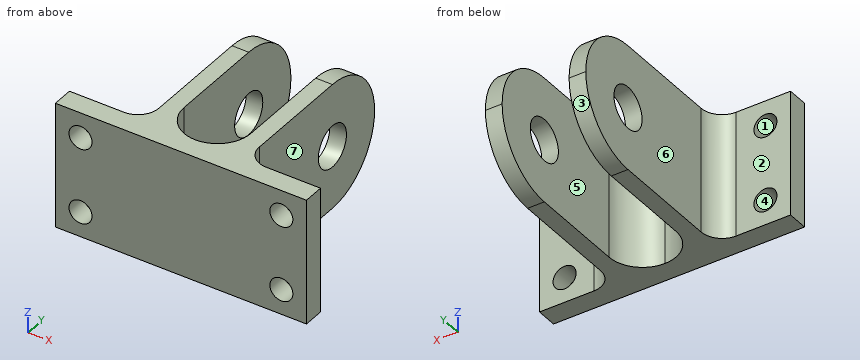
Autodesk Inventor part; units mm, degrees
ref_plane "YZ Plane" through (0, 0, 0) normal (1, 0, 0) x (0, 1, 0)
ref_plane "XZ Plane" through (0, 0, 0) normal (0, 1, 0) x (-1, 0, 0)
ref_plane "XY Plane" through (0, 0, 0) normal (0, 0, 1) x (1, 0, 0)
sketch "Sketch1" plane through (0, 0, 0) normal (0, 1, 0) x (-1, 0, 0)
  line L0 (-30, 15) -> (30, 15)
  line L1 (30, 15) -> (30, -15)
  line L2 (30, -15) -> (-30, -15)
  line L3 (-30, -15) -> (-30, 15)
  line L4 (-30, 15) -> (30, -15) construction
  line L5 (30, 15) -> (-30, -15) construction
  circle A0 centre (24, -9) radius 2.75
  circle A1 centre (24, 9) radius 2.75
  circle A2 centre (-24, 9) radius 2.75
  circle A3 centre (-24, -9) radius 2.75
  point P0 (0, 0)
  dimension "d0" = 60
  dimension "d1" = 30
  dimension "d2" = 5.5
  dimension "d3" = 5.5
  dimension "d4" = 5.5
  dimension "d5" = 5.5
  dimension "d6" = 6
  dimension "d7" = 6
  dimension "d8" = 6
  dimension "d9" = 6
  dimension "d10" = 6
  dimension "d11" = 6
  dimension "d12" = 6
  dimension "d13" = 6
extrude "Extrusion1" add sketch "Sketch1" along normal blind 5
sketch "Sketch2" plane through (0, 5, 0) normal (0, 1, 0) x (1, 0, 0)
  line L0 (8, -15) -> (-8, -15)
  line L1 (-8, -15) -> (-8, 15)
  line L2 (-8, 15) -> (8, 15)
  line L3 (8, 15) -> (8, -15)
  line L4 (8, -15) -> (-8, 15) construction
  line L5 (-8, -15) -> (8, 15) construction
  line L6 (-8, 15) -> (-12, 15)
  line L7 (-12, 15) -> (-12, -15)
  line L8 (-12, -15) -> (-8, -15)
  line L9 (-8, -15) -> (-8, 15)
  line L10 (8, -15) -> (12, -15)
  line L11 (12, -15) -> (12, 15)
  line L12 (12, 15) -> (8, 15)
  line L13 (8, 15) -> (8, -15)
  point P0 (0, 0)
  dimension "d16" = 16
  dimension "d17" = 30
  dimension "d18" = 4
  dimension "d19" = 30
  dimension "d20" = 4
extrude "Extrusion2" add sketch "Sketch2" along normal blind 46 contours L3 L12 L11 L10 | L8 L7 L6 L1
sketch "Sketch3" plane through (12, 5, 15) normal (1, 0, 0) x (0, 0, -1)
  circle A0 centre (15, 31) radius 5
  line L0 (30, 0) -> (30, 46)
  line L1 (30, -5) -> (0, -5)
  point P0 (15, -5)
  dimension "d23" = 10
  dimension "d24" = 15
  dimension "d25" = 36
extrude "Extrusion3" cut sketch "Sketch3" against normal blind 40
fillet "Fillet1" radius 15 4 edges at (10, 51, 15) (10, 51, -15) (-10, 51, -15) (-10, 51, 15)
fillet "Fillet2" radius 5 2 edges at (12, 5, 0) (-12, 5, 0)
fillet "Fillet3" radius 8 2 edges at (-8, 5, 0) (8, 5, 0)
properties part number "Custom Pneumatic Support" material "Stainless Steel"
For this review, take the finished solid that the model builds, in its own axes (mm). Face numbers are marked on the shaded views. A direction names the side the tool comes from. Coordinates: 2 decimals unless noted, no trailing zeros. Order: outer loops, then holes, each group sorted by start corner. A loop starts at its lowest first (then second) coordinate and runs counter-clockwise, first axis right, second up. Notation, with made-up numbers: (-35, 7.5) -> (-15, 7.5) arc R22 cw to (-15, 16.5) -> close; hole circle Ø8 at (32, 75.25). An arc over 180 degrees is marked (long way). Return JSON: item names as keys, results as strings.
1. We need section B-B on y = 12. Write out the cut boundary in (x, z), and give its area (3 significant figures).
Answer block:
{"outline": "(-12, -15) -> (-7.94, -15) -> (-7.94, 15) -> (-12, 15) -> close; (7.94, -15) -> (12, -15) -> (12, 15) -> (7.94, 15) -> close", "area": "244 mm²"}
2. For pin 1 Ø3 at (x, z) = (-10.5, 3.5) entering from +Y; pin 2 Ø2 at (y, z) = (16.5, -7.5) entering from +X; pin 3 Ø6.5 at (x, z) = (23, 6) entering from +Y, all flat-tipped, find the tip position at first contact; note any pin that passes through.
Answer block:
{"pin 1": "y = 50.87", "pin 2": "x = 12", "pin 3": "y = 5"}
3. Machinability: for the marked faces 4, 5, 6 and 7, which of the approach directions +Z, -Z, +X, -X, +Y, -Y give a long, thin tool a straight path to every point of the face, cutting with its end or side? Answer none if there is none.
Answer block:
{"face 4": "+Y, -Y", "face 5": "+Z, -Z, +Y", "face 6": "+Z, -Z, -X, +Y", "face 7": "+Z, -Z, +X, +Y"}
4. The part is to be moulded in two halves that separate along Z. For the marked faces 1, 2 and 3, say which applies: +Z half, -Z half, draft (parallel to the pull), parting line (faces both ways), or undercut.
Answer block:
{"face 1": "undercut", "face 2": "draft", "face 3": "-Z half"}
5. We need section C-C on z = -9. State how many separate pieces and enclosed holes the cut face has, and give its area (3 significant figures).
Answer block:
{"separate pieces": "3", "enclosed holes": "0", "area": "627 mm²"}
6. For line 1 (Z direction, x = -24, y = 3); line 2 (X direction, y = 24, z = -0.5); line 3 (X direction, y = 3, z = 7), list the stretches that pass through material, from the lowest coordinate up. Write a range as from..to.
Answer block:
{"line 1": "-15..-11.75, -6.25..6.25, 11.75..15", "line 2": "-12..-8, 8..12", "line 3": "-30..-25.89, -22.11..22.11, 25.89..30"}
7. We need section D-D on x = 24. Write out the cut boundary in (y, z), and give its area (3 significant figures).
Answer block:
{"outline": "(0, -15) -> (5, -15) -> (5, -11.75) -> (0, -11.75) -> close; (0, -6.25) -> (5, -6.25) -> (5, 6.25) -> (0, 6.25) -> close; (0, 11.75) -> (5, 11.75) -> (5, 15) -> (0, 15) -> close", "area": "95.0 mm²"}
